```python
from build123d import *

# Parameters (mm, degrees)
SKETCH1_R           = 1.5
SKETCH1_R_2         = 11.5
BOSS_EXTRUDE1_DEPTH = 5


with BuildPart() as part:
    # Sketch1 → Boss-Extrude1 (new body)
    with BuildSketch(Plane.XY):
        Polygon((0, 80), (-80, 80), (-80, 70), (-85, 70), (-85, 65), (-80, 65), (-80, 61.5), (-77, 61.5), (-77, 62.6), (-74.7, 62.6), (-74.7, 61.5), (-70, 61.5), (-70, 58.5), (-74.7, 58.5), (-74.7, 57.4), (-77, 57.4), (-77, 58.5), (-80, 58.5), (-80, 55), (-85, 55), (-85, 50), (-80, 50), (-80, 30), (-85, 30), (-85, 25), (-80, 25), (-80, 21.5), (-77, 21.5), (-77, 22.6), (-74.7, 22.6), (-74.7, 21.5), (-70, 21.5), (-70, 18.5), (-74.7, 18.5), (-74.7, 17.4), (-77, 17.4), (-77, 18.5), (-80, 18.5), (-80, 15), (-85, 15), (-85, 10), (-80, 10), (-80, 0), (0, 0), (0, 10), (5, 10), (5, 15), (0, 15), (0, 18.5), (-3, 18.5), (-3, 17.4), (-5.3, 17.4), (-5.3, 18.5), (-10, 18.5), (-10, 21.5), (-5.3, 21.5), (-5.3, 22.6), (-3, 22.6), (-3, 21.5), (0, 21.5), (0, 25), (5, 25), (5, 30), (0, 30), (0, 50), (5, 50), (5, 55), (0, 55), (0, 58.5), (-3, 58.5), (-3, 57.4), (-5.3, 57.4), (-5.3, 58.5), (-10, 58.5), (-10, 61.5), (-5.3, 61.5), (-5.3, 62.6), (-3, 62.6), (-3, 61.5), (0, 61.5), (0, 65), (5, 65), (5, 70), (0, 70), align=None)
        with Locations((-55.922, 70.922)):
            Circle(SKETCH1_R, mode=Mode.SUBTRACT)
        with Locations((-24.078, 70.922)):
            Circle(SKETCH1_R, mode=Mode.SUBTRACT)
        with Locations((-24.078, 39.078)):
            Circle(SKETCH1_R, mode=Mode.SUBTRACT)
        with Locations((-55.922, 39.078)):
            Circle(SKETCH1_R, mode=Mode.SUBTRACT)
        with Locations((-40, 55)):
            Circle(SKETCH1_R_2, mode=Mode.SUBTRACT)
    extrude(amount=BOSS_EXTRUDE1_DEPTH)


solid = part.part
```
Geometry check sheet. Reference: the model listing, model coordinates, mm. A direction names the side the tool comes from. Round coordinates to 2 decimals unless told otherwise and drop trailing zeros. Loops run counter-clockwise (first coordinate to the right, second up) from the corner with the lowest first, then second, coordinate; pieces in that order, holes last. Notation, with made-up numbers: (-29, 87.25) - (-7, 87.25) arc R24 cw to (-7, 99.25) - close; hole circle Ø4 at (-16.5, 83). An arc over 180 degrees is marked (long way). Write each question's results on one line, items separated by ' | '. Start each with the question number.
Q1. Release check for a two-part mould opening along X. For faces 1 (the flat face through (0, 23, 2)), 2 (the flat face through (-76, 57.4, 2)), 3 (the flat face through (-85, 68, 2)), 4 (the flat face through (-76, 22.6, 2)) record: +X half, -X half, draft (parallel to the pull), parting line (faces both ways), or undercut.
Q2. Cross-section at B-B on x = -40. Enter the section's corners in (y, z).
Q3. Thickness scan on line 1 (Y direction, x = -0.5, z = 0.2); line 2 (Y direction, x = -24, z = 4.5); line 3 (X direction, y = 39, z = 0.4). Record the ranges inside material, lowest first. Write a range as [from, to].
Q4. Cross-section at A-A on x = -9. Enter the section's corners in (y, z), and give its area (3 significant figures).
Q5. Access from +Z, -Z, +X, -X, +Y, -Y to the whole of each face (thin tool, end or side, straight path). Record for faces 5 (the flat face through (-82, 70, 2)), 6 (the flat face through (-2, 21.5, 2)), 7 (the flat face through (3, 70, 2)), 8 (the flat face through (-80, 63, 2)), 9 (the flat face through (-80, 5, 2)).
Q6. Gauge pin test, flat ends, axial feed: P1, Ø1.2, axis at y = 58, z = 1.5, coming from the +X side; P2, Ø2.5, axis at x = -55.922, y = 39.078, coming from the -Z side; P3, Ø2.5, axis at x = 2.5, z = 3.5, coming from the +Y side; P4, Ø2.5, axis at x = -83, z = 3, coming from the -Y side. Record the tip position at first contact, or that the pin passes through.
Q7. Cross-section at C-C on z = 3.1. State how many separate pieces and enclosed holes the cut face has, and give its area (3 significant figures).
Answers below:
1) face 1: +X half | face 2: undercut | face 3: -X half | face 4: undercut
2) outline: (0, 0) - (43.5, 0) - (43.5, 5) - (0, 5) - close; (66.5, 0) - (80, 0) - (80, 5) - (66.5, 5) - close
3) line 1: y = [0, 18.5], [21.5, 58.5], [61.5, 80] | line 2: y = [0, 37.58], [40.58, 69.42], [72.42, 80] | line 3: x = [-80, -57.42], [-54.42, -25.58], [-22.58, 0]
4) outline: (0, 0) - (18.5, 0) - (18.5, 5) - (0, 5) - close; (21.5, 0) - (58.5, 0) - (58.5, 5) - (21.5, 5) - close; (61.5, 0) - (80, 0) - (80, 5) - (61.5, 5) - close | area: 370 mm²
5) face 5: +Z, -Z, -X, +Y | face 6: +Z, -Z, +X | face 7: +Z, -Z, +X, +Y | face 8: +Z, -Z, -X | face 9: +Z, -Z, -X, -Y
6) P1: stops at x = 0 | P2: passes through | P3: stops at y = 70 | P4: stops at y = 10
7) separate pieces: 1 | enclosed holes: 5 | area: 6,020 mm²
